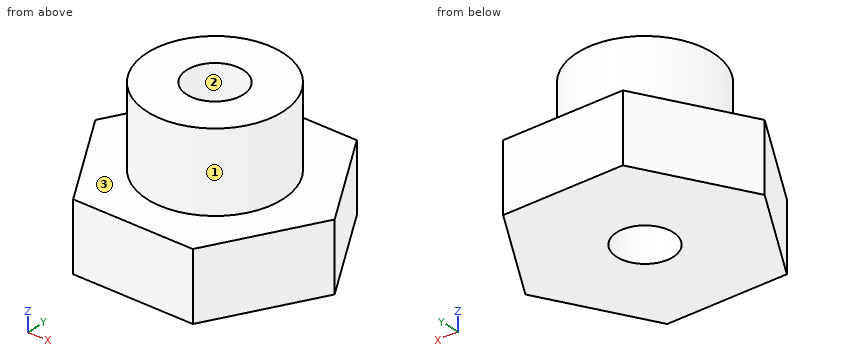
```python
from build123d import *

# Parameters (mm, degrees)
SKETCH1_R           = 6
SKETCH1_R_2         = 2.5
BOSS_EXTRUDE1_DEPTH = 6
BOSS_EXTRUDE2_START = 7
SKETCH1_3_R         = 6
SKETCH1_3_R_2       = 2.5
BOSS_EXTRUDE2_DEPTH = 7


with BuildPart() as part:
    # Sketch1 → Boss-Extrude1 (new body)
    # profile 1 of 2: a face of its own
    with BuildSketch(Plane.XY):
        Polygon((-5.196152423, -9), (5.196152423, -9), (10.392304845, 0), (5.196152423, 9), (-5.196152423, 9), (-10.392304845, 0), align=None)
        Circle(SKETCH1_R, mode=Mode.SUBTRACT)
    # profile 2 of 2: a face of its own
    with BuildSketch(Plane.XY):
        Circle(SKETCH1_R)
        Circle(SKETCH1_R_2, mode=Mode.SUBTRACT)
    extrude(amount=-BOSS_EXTRUDE1_DEPTH)

    # Sketch1_3 → Boss-Extrude2 (add)
    with BuildSketch(Plane.XY.offset(BOSS_EXTRUDE2_START)):
        Circle(SKETCH1_3_R)
        Circle(SKETCH1_3_R_2, mode=Mode.SUBTRACT)
    extrude(amount=-BOSS_EXTRUDE2_DEPTH)


solid = part.part
```
Can you work these out from the model? Positions are in its coordinate system, mm. Face numbers are marked on the shaded views. Round coordinates to 2 decimals unless told otherwise and drop trailing zeros. Loops run counter-clockwise (first coordinate to the right, second up) from the corner with the lowest first, then second, coordinate; pieces in that order, holes last. Notation, with made-up numbers: M 67.25,33 L 91.25,33 A26 ccw 91.25,56 Z; hole C 70,55.25 d11. An arc over 180 degrees is marked long. Answer as a JSON object with one key per item and string values. Group by question number.
Q1. Imagine slicing it at B-B, the plane y = -0.75. Please give me the cut outline in (x, z).
Q2. Imagine slicing it at C-C, the plane z = -4. Please give me the cut outline in (x, y), then the cut area to 3 significant figures.
Q3. Imagine slicing it at D-D, the plane y = 3.75. Please give me the cut outline in (x, z), then the cut area to 3 significant figures.
Q4. Imagine slicing it at A-A, the plane x = 0. Please give me the cut outline in (y, z).
Q5. Will these pins go through, and if not, where does the flat tip stop? pin 1 (6 mm diameter, centred on y = 5, z = -0.5, fed in from +X); pin 2 (1.5 mm diameter, centred on y = 3, z = 3.5, fed in from +X).
Q6. We'd pull the mould along X, two halves only. Please class the marked faces 1, 2 and 3: +X half, -X half, draft (parallel to the pull), parting line (faces both ways), or undercut.
Q7. Please list where these lines run through material, in increasing order: L1, parallel to Y at x = 0, z = 4; L2, parallel to Y at x = 0, z = -2.75; L3, parallel to Z at x = 1.75, y = 8.
Findings:
{
 "1": {"outline": "M -9.96,-6 L -2.38,-6 L -2.38,7 L -5.95,7 L -5.95,0 L -9.96,0 Z; M 2.38,-6 L 9.96,-6 L 9.96,0 L 5.95,0 L 5.95,7 L 2.38,7 Z"},
 "2": {"outline": "M -10.39,0 L -5.2,-9 L 5.2,-9 L 10.39,0 L 5.2,9 L -5.2,9 Z; hole C 0,0 d5", "area": "261 mm2"},
 "3": {"outline": "M -8.23,-6 L 8.23,-6 L 8.23,0 L 4.68,0 L 4.68,7 L -4.68,7 L -4.68,0 L -8.23,0 Z", "area": "164 mm2"},
 "4": {"outline": "M -9,-6 L -2.5,-6 L -2.5,7 L -6,7 L -6,0 L -9,0 Z; M 2.5,-6 L 9,-6 L 9,0 L 6,0 L 6,7 L 2.5,7 Z"},
 "5": {"pin 1": "stops at x = 9.24", "pin 2": "stops at x = 5.56"},
 "6": {"face 1": "parting line", "face 2": "undercut", "face 3": "draft"},
 "7": {"L1": "y = -6 to -2.5, 2.5 to 6", "L2": "y = -9 to -2.5, 2.5 to 9", "L3": "z = -6 to 0"}
}
